The model under review builds one solid part; all positions refer to its coordinate system, in mm. Face numbers are marked on the shaded views. A direction names the side the tool comes from. Coordinates: 2 decimals unless noted, no trailing zeros. Order: outer loops, then holes, each group sorted by start corner. A loop starts at its lowest first (then second) coordinate and runs counter-clockwise, first axis right, second up. Notation, with made-up numbers: (50, -15) -> (61, -15) arc R18 cw to (61, 14) -> close; hole circle Ø10 at (87.5, 22.25). An arc over 180 degrees is marked (long way). Put each result on its own line as item: value.
from build123d import *

# Parameters (mm, degrees)
F1_DEPTH = 4
F4_DEPTH = 25
F5_R     = 0.5
F6_DEPTH = 12.5


with BuildPart() as f1:
    # F0 (on Front) → F1 (new body, symmetric)
    with BuildSketch(Plane.XZ):
        with BuildLine():
            Line((-2.5, 16), (2.5, 16))
            ThreePointArc((2.5, 16), (0, 18.5), (-2.5, 16))
        make_face()
        with BuildLine():
            ThreePointArc((-2.5, 16), (0, 13.5), (2.5, 16))
            Line((2.5, 16), (-2.5, 16))
        make_face()
    extrude(amount=F1_DEPTH, both=True)

    # F3 (on offset) → F4 (cut)
    with BuildSketch(Plane.XZ.offset(4)):
        with BuildLine():
            ThreePointArc((0, 15.5), (0.3535533906, 15.6464466094), (0.5, 16))
            ThreePointArc((0.5, 16), (-0.3535533906, 16.3535533906), (0, 15.5))
        make_face()
    extrude(amount=-F4_DEPTH, mode=Mode.SUBTRACT)

    # F5 (on Front) → F6 (join, symmetric)
    with BuildSketch(Plane.XZ):
        with Locations((0, 16)):
            Circle(F5_R)
    extrude(amount=F6_DEPTH, both=True)


solid = f1.part
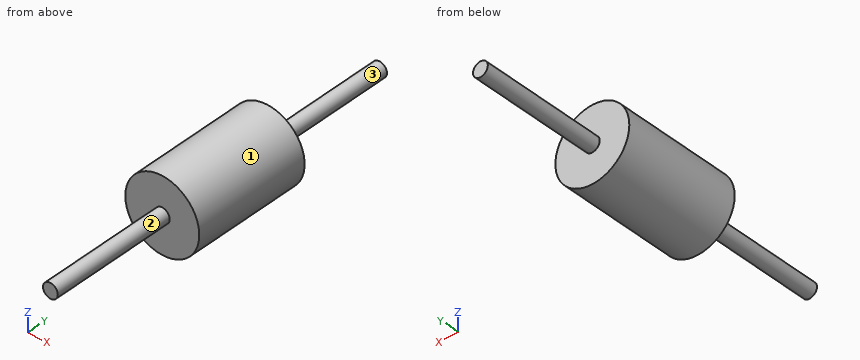
Item 1: For the marked faces 1, 2 and 3, list the 3-axis set-ups (+Z, -Z, +X, -X, +Y, -Y) from which the entire face can be reached by the end or side of a thin tool; tool diameter is ignored.
Answers below:
face 1: +Y, -Y
face 2: -Y
face 3: +Y
Item 2: For pin 1 Ø3 at (x, y) = (-0.5, -8.5) entering from +Z; pin 2 Ø2 at (x, z) = (0, 15) entering from +Y; pin 3 Ø1 at (y, z) = (8.5, 16) entering from +X, all flat-tipped, find the tip position at first contact; note any pin that passes through.
Answers below:
pin 1: z = 16.5
pin 2: y = 12.5
pin 3: x = 0.5
Item 3: For line 1 (Y direction, x = -0.3, z = 16.65); line 2 (Z direction, x = -0.3, y = 3.75); line 3 (X direction, y = 3.5, z = 15.4), list the stretches that pass through material, from the lowest coordinate up. Write a range as from..to.
Answers below:
line 1: -4..4
line 2: 13.52..18.48
line 3: -2.43..2.43
Item 4: Consider section A-A on z = 16. Write out the cut boundary in (x, y).
Answers below:
outline: (-2.5, -4) -> (-0.5, -4) -> (-0.5, -12.5) -> (0.5, -12.5) -> (0.5, -4) -> (2.5, -4) -> (2.5, 4) -> (0.5, 4) -> (0.5, 12.5) -> (-0.5, 12.5) -> (-0.5, 4) -> (-2.5, 4) -> close
Item 5: Consider section B-B on x = 0. Write out the cut boundary in (y, z), and give its area (3 significant figures).
Answers below:
outline: (-12.5, 15.5) -> (-4, 15.5) -> (-4, 13.5) -> (4, 13.5) -> (4, 15.5) -> (12.5, 15.5) -> (12.5, 16.5) -> (4, 16.5) -> (4, 18.5) -> (-4, 18.5) -> (-4, 16.5) -> (-12.5, 16.5) -> close
area: 57.0 mm^2
Item 6: Consider section C-C on y = 10.5. Write out the cut boundary in (x, z).
Answers below:
outline: circle Ø1 at (0, 16)
Item 7: Consider section D-D on y = 2.25. Write out the cut boundary in (x, z).
Answers below:
outline: circle Ø5 at (0, 16)
